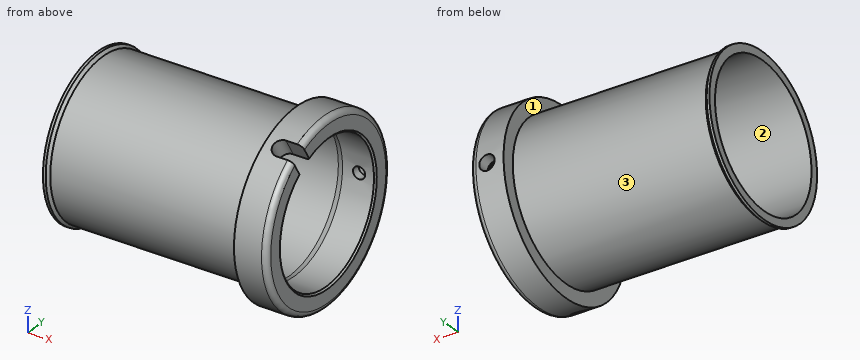
from build123d import *

# Parameters (mm, degrees)
SKETCH031_R           = 2.8
POCKET195_DEPTH       = 4.5
SKETCH032_R           = 2.2
POCKET196_DEPTH       = 284.142395
POLARPATTERN008_COUNT = 2
POLARPATTERN008_ANGLE = 120
POCKET197_DEPTH       = 20.679838
CHAMFER001_SIZE       = 0.6


with BuildPart() as part:
    # Sketch022 → Revolution001 (revolve)
    with BuildSketch(Plane.XY):
        with BuildLine():
            Line((0, 26), (70.133975, 26))
            Line((70.133975, 26), (72, 25.5))
            Line((72, 25.5), (84, 25.5))
            Line((84, 31), (84, 25.5))
            ThreePointArc((84, 31), (83.414214, 32.414214), (82, 33))
            Line((72, 33), (82, 33))
            Line((72, 28), (72, 33))
            Line((2, 28), (72, 28))
            Line((1, 29), (2, 28))
            Line((0, 29), (1, 29))
            Line((0, 26), (0, 29))
        make_face()
    revolve(axis=Axis((0, 0, 0), (1, 0, 0)))

    # Sketch031 (on DatumPlane) → Pocket195 (cut)
    with BuildSketch(Plane(origin=(78, 33, 0), x_dir=(-1, 0, 0), z_dir=(0, 1, 0))):
        Circle(SKETCH031_R)
    pocket195 = extrude(amount=-POCKET195_DEPTH, mode=Mode.SUBTRACT)

    # Sketch032 (on DatumPlane) → Pocket196 (cut, through all)
    with BuildSketch(Plane(origin=(78, 0, 0), x_dir=(1, 0, 0), z_dir=(0, -1, 0))):
        Circle(SKETCH032_R)
    pocket196 = extrude(amount=-POCKET196_DEPTH, mode=Mode.SUBTRACT)

    # PolarPattern008: Pocket195, Pocket196 ×2 about axis
    polarpattern008_axis = Axis((0, 0, 0), (-1, 0, 0))
    for i in range(1, POLARPATTERN008_COUNT):
        add(pocket195.rotate(polarpattern008_axis, i * POLARPATTERN008_ANGLE / (POLARPATTERN008_COUNT - 1)), mode=Mode.SUBTRACT)
        add(pocket196.rotate(polarpattern008_axis, i * POLARPATTERN008_ANGLE / (POLARPATTERN008_COUNT - 1)), mode=Mode.SUBTRACT)

    # Sketch146 (on DatumPlane) → Pocket197 (cut, through all)
    with BuildSketch(Plane(origin=(78, -12.2, 21.13102), x_dir=(1, 0, 0), z_dir=(0, 0.5, -0.866025))):
        with BuildLine():
            Line((7, 3), (0, 3))
            ThreePointArc((0, 3), (-3, 0), (0, -3))
            Line((0, -3), (7, -3))
            Line((7, -3), (7, 3))
        make_face()
    extrude(amount=-POCKET197_DEPTH, mode=Mode.SUBTRACT)

    # Chamfer001
    chamfer001_edges = [part.edges().sort_by_distance(p)[0] for p in [
        (84, 14.029144, 21.293969),
        (84, -11.426546, -22.79658),
    ]]
    chamfer(chamfer001_edges, length=CHAMFER001_SIZE)


with BuildPart() as part_1:
    # Body007 placement: moved
    add(part.part.moved(Location((110, 0, 835))))


solid = part_1.part
Can you work these out from the model? Positions are in its coordinate system, mm. Face numbers are marked on the shaded views. Coordinates: 2 decimals unless noted, no trailing zeros. Write each loop counter-clockwise with the first axis right and the second up, starting at its lowest first coordinate (ties: lowest second). Pieces come first, ordered by that corner, then holes.
Q1. Please list where these lines run through material, in increasing order: L1, parallel to X at y = 29.8, z = 835; L2, parallel to Z at x = 186.5, y = 0; L3, parallel to X at y = 24, z = 818.
Results found:
L1: x = 182 to 185.2, 190.8 to 194
L2: z = 802 to 809.5, 860.5 to 868
L3: x = 182 to 194
Q2. Imagine slicing it at A-A, the plane y = 0. List the corners of the cut face in (x, z) for me, plus the area to 3 significant figures.
Results found:
outline: (110, 806) - (111, 806) - (112, 807) - (182, 807) - (182, 802) - (192, 802) arc R2 ccw to (194, 804) - (194, 808.9) - (193.4, 809.5) - (182, 809.5) - (180.13, 809) - (110, 809) - close; (110, 861) - (180.13, 861) - (182, 860.5) - (193.4, 860.5) - (194, 861.1) - (194, 866) arc R2 ccw to (192, 868) - (182, 868) - (182, 863) - (112, 863) - (111, 864) - (110, 864) - close
area: 470 mm2
Q3. Imagine slicing it at C-C, the plane x = 142. List the corners of the cut face in (y, z) for me, plus the area to 3 significant figures.
Results found:
outline: circle Ø56 at (0, 835); hole circle Ø52 at (0, 835)
area: 339 mm2
Q4. If we mould it in two halves opening along Z, with no side actions, what happens to the marked faces 1, 2 and 3? For each: +Z half, -Z half, draft (parallel to the pull), parting line (faces both ways), or undercut.
Results found:
face 1: draft
face 2: undercut
face 3: parting line
Q5. For P1, Ø3, axis at x = 189.5, z = 836, coming from the +Y side; P2, Ø10, axis at x = 135, y = -4.5, coming from the +Z side; P3, Ø4, axis at x = 144, y = 11.5, coming from the -Z side; P4, Ø3, axis at x = 142.5, z = 831.5, coming from the +Y side, each with a flat end and sliding along its axis, tell me the tip position at first contact or that it passes through.
Results found:
P1: stops at y = 33
P2: stops at z = 863
P3: stops at z = 808.66
P4: stops at y = 27.93
Q6. Imagine slicing it at B-B, the plane z = 835. Count the separate pieces of the cut face and the enclosed holes in it, plus the area to 3 significant figures.
Results found:
separate pieces: 3
enclosed holes: 0
area: 431 mm2
